Here's the drawing with two shaded views (mm, measured from the low corner). I have some questions. Give positions to 0.01 mm unless a question says otherwise; leave off trailing zeros. Write each loop counter-clockwise with the first axis right and the second up, starting at its lowest first coordinate (ties: lowest second). Pieces come first, ordered by that corner, then holes.
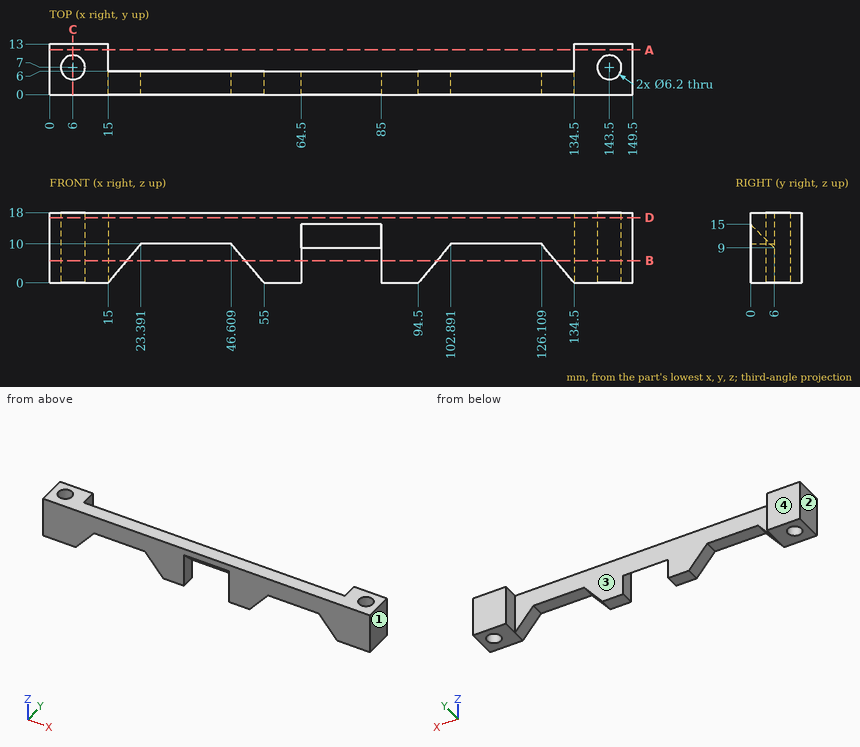
1) Suppose I cut it at A-A on y = 11.5. Write out the boundary of the cut face in (x, z).
Values follow:
outline: (0, 0) - (15, 0) - (15, 18) - (0, 18) - close; (134.5, 0) - (149.5, 0) - (149.5, 18) - (134.5, 18) - close
2) For pin 1 Ø3 at (x, y) = (38, 3) entering from -Z; pin 2 Ø9 at (x, z) = (98, 11) entering from +Y, each with a flat end and sliding along its axis, tell me the tip position at first contact or that it passes through.
Values follow:
pin 1: stops at z = 10
pin 2: stops at y = 6
3) Suppose I cut it at B-B on z = 5.75. Write out the boundary of the cut face in (x, y).
Values follow:
outline: (0, 0) - (19.82, 0) - (19.82, 6) - (15, 6) - (15, 13) - (0, 13) - close; (50.18, 0) - (64.5, 0) - (64.5, 6) - (50.18, 6) - close; (85, 0) - (99.32, 0) - (99.32, 6) - (85, 6) - close; (129.68, 0) - (149.5, 0) - (149.5, 13) - (134.5, 13) - (134.5, 6) - (129.68, 6) - close; hole circle Ø6.2 at (6, 7); hole circle Ø6.2 at (143.5, 7)
4) Please list where these lines run through material, in increasing order: L1, parallel to Y at x = 6, z = 5; L2, parallel to X at y = 1, z = 11; L3, parallel to X at y = 9, z = 15.75.
Values follow:
L1: y = 0 to 3.9, 10.1 to 13
L2: x = 0 to 64.5, 85 to 149.5
L3: x = 0 to 3.63, 8.37 to 15, 134.5 to 141.13, 145.87 to 149.5
5) Suppose I cut it at C-C on x = 6. Write out the boundary of the cut face in (y, z), plus the area to 3 significant figures.
Values follow:
outline: (0, 0) - (3.9, 0) - (3.9, 18) - (0, 18) - close; (10.1, 0) - (13, 0) - (13, 18) - (10.1, 18) - close
area: 122 mm2
6) If we mould it in two halves opening along X, with no side actions, what happens to the marked faces 1, 2, 3 and 4? For each: +X half, -X half, draft (parallel to the pull), parting line (faces both ways), or undercut.
Values follow:
face 1: +X half
face 2: -X half
face 3: undercut
face 4: draft
7) Suppose I cut it at D-D on z = 16.75. Write out the boundary of the cut face in (x, y), plus the area to 3 significant figures.
Values follow:
outline: (0, 0) - (149.5, 0) - (149.5, 13) - (134.5, 13) - (134.5, 6) - (15, 6) - (15, 13) - (0, 13) - close; hole circle Ø6.2 at (6, 7); hole circle Ø6.2 at (143.5, 7)
area: 1,050 mm2
